CAD build for the part. Positions are in the model's coordinates, mm. Face numbers are marked on the shaded views. A direction names the side the tool comes from. Give positions to 0.01 mm unless a question says otherwise; leave off trailing zeros. Loops run counter-clockwise (first coordinate to the right, second up) from the corner with the lowest first, then second, coordinate; pieces in that order, holes last. Notation, with made-up numbers: (16, 34) -> (62, 34) arc R33 ccw to (62, 65) -> close; hole circle Ø2 at (14, -18). An arc over 180 degrees is marked (long way). Use one line per item in the form item = value.
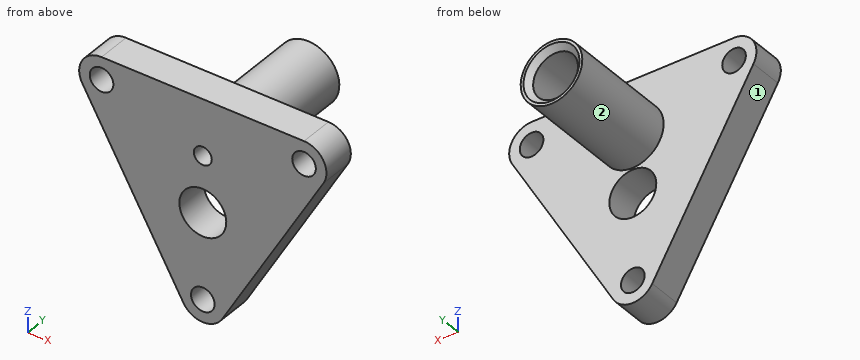
```python
from build123d import *

# Parameters (mm, degrees)
SKETCH1_R           = 1.054
BOSS_EXTRUDE1_DEPTH = 3
SKETCH2_R           = 0.8
SKETCH2_R_2         = 2.0955
CUT_EXTRUDE1_DEPTH  = 23.736281859
SKETCH3_R           = 2.75
BOSS_EXTRUDE2_DEPTH = 10
CUT_EXTRUDE2_REACH  = 26.656
SKETCH4_R           = 2
CHAMFER1_SIZE       = 2
CHAMFER1_SIZE2      = 0.727940469
CHAMFER2_SIZE       = 0.5


with BuildPart() as part:
    # Sketch1 → Boss-Extrude1 (new body)
    with BuildSketch(Plane(origin=(0, 0, 0), x_dir=(1, 0, 0), z_dir=(0, 1, 0))):
        with BuildLine():
            Line((0, 0), (9.035898385, 0))
            ThreePointArc((9.035898385, 0), (10.767949192, 1), (10.767949192, 3))
            Line((10.767949192, 3), (1.732050808, 18.650635095))
            ThreePointArc((1.732050808, 18.650635095), (0, 19.650635095), (-1.732050808, 18.650635095))
            Line((-1.732050808, 18.650635095), (-10.767949192, 3))
            ThreePointArc((-10.767949192, 3), (-10.767949192, 1), (-9.035898385, 0))
            Line((-9.035898385, 0), (0, 0))
        make_face()
        with Locations(Location((0, 17.650635095, 0), (0, 0, 270))):
            Circle(SKETCH1_R, mode=Mode.SUBTRACT)
        with Locations(Location((-9.035898385, 2, 0), (0, 0, 270))):
            Circle(SKETCH1_R, mode=Mode.SUBTRACT)
        with Locations(Location((9.035898385, 2, 0), (0, 0, 270))):
            Circle(SKETCH1_R, mode=Mode.SUBTRACT)
    extrude(amount=BOSS_EXTRUDE1_DEPTH)

    # Sketch2 → Cut-Extrude1 (cut, through all)
    with BuildSketch(Plane(origin=(0, 3, 0), x_dir=(1, 0, 0), z_dir=(0, 1, 0))):
        with Locations(Location((0, 5, 0), (0, 0, 270))):
            Circle(SKETCH2_R)
        with Locations(Location((0, 10, 0), (0, 0, 270))):
            Circle(SKETCH2_R_2)
    extrude(amount=-CUT_EXTRUDE1_DEPTH, mode=Mode.SUBTRACT)

    # Sketch3 → Boss-Extrude2 (add)
    with BuildSketch(Plane(origin=(0, 3, 0), x_dir=(1, 0, 0), z_dir=(0, 1, 0))):
        with Locations(Location((0, 5, 0), (0, 0, 270))):
            Circle(SKETCH3_R)
    extrude(amount=BOSS_EXTRUDE2_DEPTH)

    # Sketch4 → Cut-Extrude2 (cut, up to next)
    with BuildSketch(Plane(origin=(0, 3, 0), x_dir=(1, 0, 0), z_dir=(0, 1, 0)), mode=Mode.PRIVATE) as cut_extrude2_sk1:
        with Locations(Location((0, 5, 0), (0, 0, 270))):
            Circle(SKETCH4_R)
    cut_extrude2_tool1 = extrude(cut_extrude2_sk1.sketch, amount=CUT_EXTRUDE2_REACH, mode=Mode.PRIVATE) & part.part
    add(cut_extrude2_tool1.solids().sort_by_distance((0, 3, -5))[0], mode=Mode.SUBTRACT)

    # Chamfer1
    chamfer1_edges = [part.edges().sort_by_distance(p)[0] for p in [
        (0, 3, -7),
    ]]
    chamfer1_side = [part.faces().sort_by_distance(p)[0] for p in [
        (0, 8, -7),
    ]]
    chamfer(chamfer1_edges, length=CHAMFER1_SIZE, length2=CHAMFER1_SIZE2, reference=chamfer1_side[0])

    # Chamfer2
    chamfer2_edges = [part.edges().sort_by_distance(p)[0] for p in [
        (0, 13, -7),
    ]]
    chamfer(chamfer2_edges, length=CHAMFER2_SIZE)


solid = part.part
```
1. Drop flat-ended pins along their axis: P1, Ø1, axis at x = -4.5, z = -4, coming from the +Y side; P2, Ø6, axis at x = -1, y = 7, coming from the +Z side; P3, Ø2, axis at y = 1.5, z = -11.5, coming from the +X side; P4, Ø4, axis at y = 10.5, z = -10, coming from the -X side. Give the stop position or say it passes through.
Result sheet:
P1 = 3
P2 = -2.25
P3 = 6.44
P4 = through
2. Cut at B-B, the plane y = 2. Write the cut outline in (x, z).
Result sheet:
outline = (-10.77, -3) -> (-1.73, -18.65) arc R2 ccw to (1.73, -18.65) -> (10.77, -3) arc R2 ccw to (9.04, 0) -> (-9.04, 0) arc R2 ccw to start; hole circle Ø2.11 at (-9.04, -2); hole circle Ø4.19 at (0, -10); hole circle Ø2.11 at (0, -17.65); hole circle Ø1.6 at (0, -5); hole circle Ø2.11 at (9.04, -2)
3. Cut at C-C, the plane y = 11. Write the cut outline in (x, z).
Result sheet:
outline = circle Ø5.5 at (0, -5); hole circle Ø4 at (0, -5)
4. Tool access for the marked faces 1 and 2: list every direction of +Z, -Z, +X, -X, +Y, -Y with a clear straight run to the whole face (end or side of a thin tool).
Result sheet:
face_1 = -Z, -X, +Y, -Y
face_2 = +Y
5. Cut at D-D, the plane z = -10. Write the cut outline in (x, y).
Result sheet:
outline = (-6.73, 0) -> (-2.1, 0) -> (-2.1, 3) -> (-6.73, 3) -> close; (2.1, 0) -> (6.73, 0) -> (6.73, 3) -> (2.1, 3) -> close
6. Cut at A-A, the plane z = -5. Write the cut outline in (x, y).
Result sheet:
outline = (-9.61, 0) -> (-0.8, 0) -> (-0.8, 3) -> (-1.27, 3) -> (-2, 5) -> (-2, 12.5) -> (-2.5, 13) -> (-2.75, 13) -> (-2.75, 3) -> (-9.61, 3) -> close; (0.8, 0) -> (9.61, 0) -> (9.61, 3) -> (2.75, 3) -> (2.75, 13) -> (2.5, 13) -> (2, 12.5) -> (2, 5) -> (1.27, 3) -> (0.8, 3) -> close
7. Drill centre lines: line 1 (X direction, y = 1, z = -2); line 2 (Y direction, x = -7.25, z = -1); line 3 (X direction, y = 7.5, z = -6.5). Where is each one in solid material? Low to high.
Result sheet:
line_1 = -11.04 to -10.09, -7.98 to 7.98, 10.09 to 11.04
line_2 = 0 to 3
line_3 = -2.3 to -1.32, 1.32 to 2.3
